Here's how the part is built. I have some questions about the finished solid (model axes, mm). Face numbers are marked on the shaded views. Coordinates: 2 decimals unless noted, no trailing zeros. Loops run counter-clockwise (first coordinate to the right, second up) from the corner with the lowest first, then second, coordinate; pieces in that order, holes last. Notation, with made-up numbers: (8.25, -10.75) -> (42.25, -10.75) arc R25 cw to (42.25, 12.25) -> close; hole circle Ø4 at (-31.75, -10). An arc over 180 degrees is marked (long way). Answer as a JSON object with one key per item and string values. Group by question number.
1) If we mould it in two halves opening along X, with no side actions, what happens to the marked faces 1, 2 and 3? For each: +X half, -X half, draft (parallel to the pull), parting line (faces both ways), or undercut.
2) I'm going to push flat-ended pins straight in: pin 1 (1.5 mm diameter, centred on x = 3.5, z = 2, fed in from +Y); pin 2 (2 mm diameter, centred on x = 3.5, z = -1, fed in from -Y). Where does each tip first touch, or does it pass through?
3) I want a section at A-A (x = 10). Write out the boundary of the cut face in (y, z).
4) I need wall thicknesses on probe 1 along Z at (x, y) = (7, 0.15); probe 2 along Z at (x, y) = (-9, 1.1) (3 decimals). Which ranges of each line are inside material? Lowest first, please. Write a range as [from, to].
Autodesk Inventor part; units mm, degrees
ref_plane "YZ Plane" through (0, 0, 0) normal (1, 0, 0) x (0, 1, 0)
ref_plane "XZ Plane" through (0, 0, 0) normal (0, 1, 0) x (-1, 0, 0)
ref_plane "XY Plane" through (0, 0, 0) normal (0, 0, 1) x (1, 0, 0)
sketch "Sketch1" plane through (0, 0, 0) normal (1, 0, 0) x (0, 1, 0)
  circle A0 centre (0, 0) radius 2.5
  dimension "d0" = 5
extrude "Extrusion1" add sketch "Sketch1" along normal blind 20
sketch "Sketch2" plane through (20, 0, 0) normal (1, 0, 0) x (0, 0, -1)
  circle A0 centre (0, 0) radius 3
  dimension "d3" = 6
extrude "Extrusion2" add sketch "Sketch2" along normal blind 2
chamfer "Chamfer1" distance 1 angle 45 1 edges at (22, 0, 3)
sketch "Sketch4" plane through (0, 0, 0) normal (-1, 0, 0) x (0, 0, 1)
  circle A0 centre (0, 0) radius 2.5
extrude "Extrusion4" add sketch "Sketch4" along normal blind 15
properties part number "Motor Shaft"
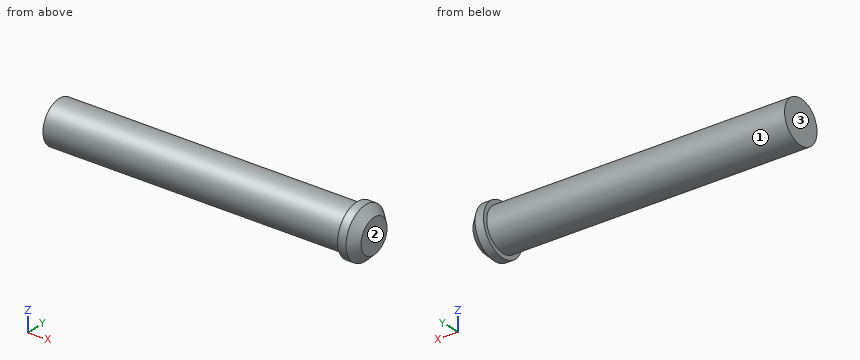
Determined:
{
 "1": {"face 1": "draft", "face 2": "+X half", "face 3": "-X half"},
 "2": {"pin 1": "y = 2.17", "pin 2": "y = -2.5"},
 "3": {"outline": "circle Ø5 at (0, 0)"},
 "4": {"probe 1": "[-2.5, 2.5]", "probe 2": "[-2.245, 2.245]"}
}
